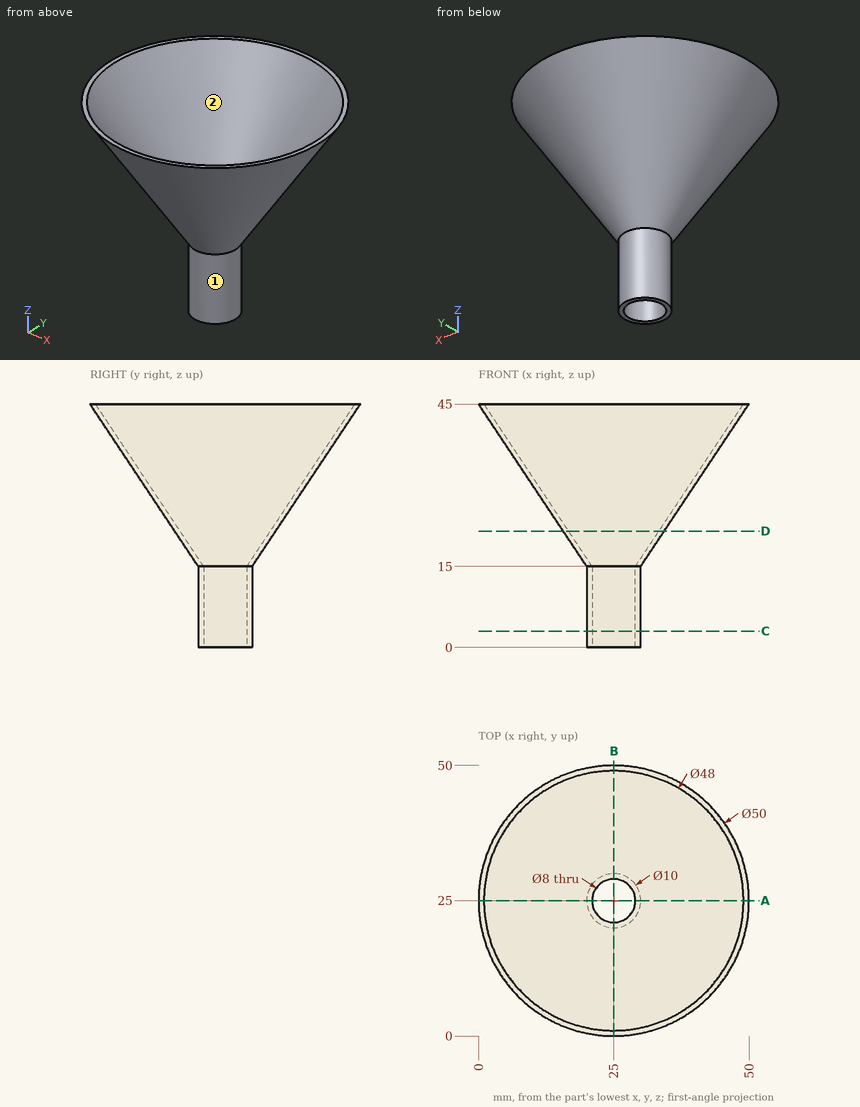
Can you work these out from the drawing? Everything is in mm from the part's minimum corner. A direction names the side the tool comes from. Coordinates: 2 decimals unless noted, no trailing zeros. Order: outer loops, then holes, each group sorted by start corner. A loop starts at its lowest first (then second) coordinate and runs counter-clockwise, first axis right, second up. Notation, with made-up numbers: (25, 23.5) -> (51, 23.5) arc R21 cw to (51, 56.5) -> close; hole circle Ø8 at (26.25, 81.5). An arc over 180 degrees is marked (long way). Use one line per item in the form item = value.
Q1. Imagine slicing it at D-D, the plane z = 21.5. List the corners of the cut face in (x, y) for me.
From the geometry:
outline = circle Ø18.67 at (25, 25); hole circle Ø16.67 at (25, 25)
Q2. I need wall thicknesses on L1, parallel to Y at x = 25, z = 6; L2, parallel to Y at x = 11.5, z = 36.5; L3, parallel to Z at x = 31.5, y = 16. Which ranges of each line are inside material? Lowest first, please.
From the geometry:
L1 = 20 to 21, 29 to 30
L2 = 11.16 to 12.6, 37.4 to 38.84
L3 = 24.15 to 25.65
Q3. Imagine slicing it at C-C, the plane z = 3. List the corners of the cut face in (x, y) for me.
From the geometry:
outline = circle Ø10 at (25, 25); hole circle Ø8 at (25, 25)
Q4. Imagine slicing it at A-A, the plane y = 25. List the corners of the cut face in (x, z) for me, then the cut area to 3 significant figures.
From the geometry:
outline = (0, 45) -> (20, 15) -> (20, 0) -> (21, 0) -> (21, 15) -> (1, 45) -> close; (29, 0) -> (30, 0) -> (30, 15) -> (50, 45) -> (49, 45) -> (29, 15) -> close
area = 90.0 mm²
Q5. Will these pins go through, and if not, where does the flat tip stop? P1, Ø13, axis at x = 25, y = 25, coming from the +Z side; P2, Ø8, axis at y = 33, z = 29.5, coming from the -X side; P3, Ø10, axis at x = 25.5, y = 7, coming from the +Z side; P4, Ø12, axis at x = 37.5, z = 6.5, coming from the -Y side.
From the geometry:
P1 = 18.75
P2 = 9.12
P3 = 43.51
P4 = through
Q6. Which directions (+Z, -Z, +X, -X, +Y, -Y) give clear straight access to the entire face, cutting with the end or side of a thin tool? Please do the marked faces 1 and 2.
From the geometry:
face_1 = -Z
face_2 = +Z
